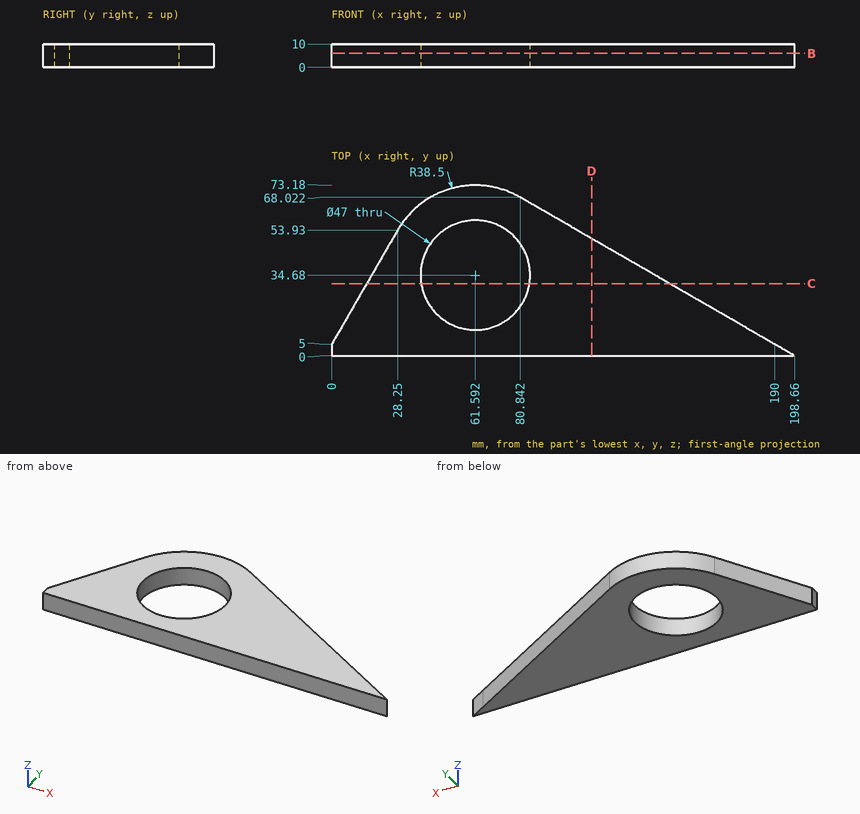
Study the drawing (mm; zero at the part's minimum x, y, z) and answer. Coordinates: 2 decimals unless noted, no trailing zeros. Order: outer loops, then holes, each group sorted by start corner. A loop starts at its lowest first (then second) coordinate and runs counter-clockwise, first axis right, second up. Notation, with made-up numbers: (40, -6) -> (63, -6) arc R32 ccw to (63, 26) -> close; hole circle Ø7 at (41, 28.25). An arc over 180 degrees is marked (long way). Answer in a Markdown table with one row per item. Add a question column.
Item 1: Find section D-D (x = 111.5). Write down the section's boundary in (y, z), then the cut area to 3 significant figures.
Item 2: Find the intervals of material crossed by L1, parallel to X at y = 37.5, z = 3 (1 decimal); L2, parallel to Y at x = 59.5, z = 7.75; L3, parallel to X at y = 39.5, z = 5.5 (1 decimal), in increasing order. Write a range as from..to.
Item 3: Find section C-C (y = 31). Write down the section's boundary in (x, z).
Item 4: Find section B-B (z = 6). Write down the section's boundary in (x, y).
Item 5: Each of these flat-tipped pins is pushed along its axis until it touches: P1, Ø1.5, axis at y = 34.5, z = 5.5, coming from the -X side; P2, Ø4, axis at y = 60.5, z = 3.5, coming from the -X side (1 decimal); P3, Ø6, axis at x = 173.5, z = 6.5, coming from the +Y side. Where does it stop, or does it pass through?
Result set:
| question | item | result |
|---|---|---|
| 1 | outline | (0, 0) -> (50.32, 0) -> (50.32, 10) -> (0, 10) -> close |
| 1 | area | 503 mm² |
| 2 | L1 | x = 18.8..38.3, 84.9..133.7 |
| 2 | L2 | y = 0..11.27, 58.09..73.12 |
| 2 | L3 | x = 19.9..38.6, 84.6..130.2 |
| 3 | outline | (15.01, 0) -> (38.38, 0) -> (38.38, 10) -> (15.01, 10) -> close; (84.8, 0) -> (144.97, 0) -> (144.97, 10) -> (84.8, 10) -> close |
| 4 | outline | (0, 0) -> (198.66, 0) -> (80.84, 68.02) arc R38.5 ccw to (28.25, 53.93) -> (0, 5) -> close; hole circle Ø47 at (61.59, 34.68) |
| 5 | P1 | stops at x = 16.6 |
| 5 | P2 | stops at x = 31.3 |
| 5 | P3 | stops at y = 16.26 |
